The model under review builds one solid part; all positions refer to its coordinate system, in mm. A direction names the side the tool comes from. Give positions to 0.01 mm unless a question says otherwise; leave off trailing zeros. Order: outer loops, then holes, each group sorted by start corner. A loop starts at its lowest first (then second) coordinate and runs counter-clockwise, first axis right, second up. Notation, with made-up numbers: (54.5, 1.25) - (110.5, 1.25) arc R21 cw to (110.5, 20.25) - close; hole circle Ø6 at (39, 53.25). An arc over 180 degrees is marked (long way). Put each result on its own line as item: value.
```python
from build123d import *

# Parameters (mm, degrees)
F1_DEPTH = 6
F0_R     = 1.5
F2_W     = 12.7708302005
F2_H     = 12
F3_DEPTH = 3
F4_R     = 3
F6_DEPTH = 4
F7_D     = 3.3


with BuildPart() as f1:
    # F0 (on Top) → F1 (new body)
    with BuildSketch(Plane.XY):
        with BuildLine():
            ThreePointArc((2.7708302005, -1.15), (-3, 0), (2.7708302005, 1.15))
            Line((2.7708302005, 1.15), (6.7708302005, 1.15))
            Line((6.7708302005, 1.15), (6.7708302005, 6))
            Line((6.7708302005, 6), (-6, 6))
            Line((-6, 6), (-6, 0))
            Line((-6, 0), (-6, -6))
            Line((-6, -6), (6.7708302005, -6))
            Line((6.7708302005, -6), (6.7708302005, -1.15))
            Line((6.7708302005, -1.15), (2.7708302005, -1.15))
        make_face()
    extrude(amount=F1_DEPTH)



with BuildPart() as f1b:
    # F0 (on Top) → F1, piece 2 (new body)
    with BuildSketch(Plane.XY):
        Circle(F0_R)
    extrude(amount=F1_DEPTH)


with BuildPart() as f1_1:
    add(f1.part)

    add(f1b.part)  # F3 merges F1b
    # F2 (on face) → F3 (join)
    with BuildSketch(Plane(origin=(0, 0, 0), x_dir=(1, 0, 0), z_dir=(0, 0, -1))):
        with Locations((0.3854151002, 0)):
            Rectangle(F2_W, F2_H)
    extrude(amount=F3_DEPTH)

    # F4
    f4_edges = [f1_1.edges().sort_by_distance(p)[0] for p in [
        (2.77083, -1.15, 3),
        (2.77083, 1.15, 3),
    ]]
    fillet(f4_edges, radius=F4_R)

    # F5 (on face) → F6 (join)
    with BuildSketch(Plane(origin=(-6, 0, 0), x_dir=(0, -1, 0), z_dir=(-1, 0, 0))):
        with BuildLine():
            Line((-6, -3), (-6, 6))
            Line((-6, 6), (-10, 6))
            ThreePointArc((-10, 6), (-13.1819805153, 4.6819805153), (-14.5, 1.5))
            ThreePointArc((-14.5, 1.5), (-13.1819805153, -1.6819805153), (-10, -3))
            Line((-10, -3), (-6, -3))
        make_face()
        with BuildLine():
            Line((10, 6), (6, 6))
            Line((6, 6), (6, -3))
            Line((6, -3), (10, -3))
            ThreePointArc((10, -3), (13.1819805153, -1.6819805153), (14.5, 1.5))
            ThreePointArc((14.5, 1.5), (13.1819805153, 4.6819805153), (10, 6))
        make_face()
    extrude(amount=-F6_DEPTH)

    # F7 (through all)
    with Locations(Plane(origin=(-6, 0, 0), x_dir=(0, -1, 0), z_dir=(-1, 0, 0))):
        with Locations((-10, 1.5), (10, 1.5)):
            Hole(F7_D / 2)


solid = f1_1.part
```
(1) Take a section at D-D, the plane x = 0. Write out the cut boundary in (y, z).
The answers:
outline: (-6, -3) - (6, -3) - (6, 6) - (3, 6) - (3, 0) - (1.5, 0) - (1.5, 6) - (-1.5, 6) - (-1.5, 0) - (-3, 0) - (-3, 6) - (-6, 6) - close
(2) Take a section at C-C, the plane x = -4. Write out the cut boundary in (y, z).
The answers:
outline: (-10, -3) - (10, -3) arc R4.5 ccw to (10, 6) - (-10, 6) arc R4.5 ccw to start; hole circle Ø3.3 at (-10, 1.5); hole circle Ø3.3 at (10, 1.5)
(3) For faces 1 (the flat face through (6, 1.15, 3)), 2 (the flat face through (-2, -8, 2)), 3 (the flat face through (-2, 8, 3)), list the 3-axis set-ups (+Z, -Z, +X, -X, +Y, -Y) from which the entire face can be reached by the end or side of a thin tool; tool diameter is ignored.
The answers:
face 1: +Z, +X
face 2: +Z, -Z, +X, -Y
face 3: +Z, -Z, +X, +Y
(4) Take a section at B-B, the plane y = -10.75. Write out the cut boundary in (x, z).
The answers:
outline: (-6, -2.94) - (-2, -2.94) - (-2, 0.03) - (-6, 0.03) - close; (-6, 2.97) - (-2, 2.97) - (-2, 5.94) - (-6, 5.94) - close
(5) Take a section at A-A, the plane z = 5.25. Write out the cut boundary in (x, y) (3 decimals).
The answers:
outline: (-6, -12.487) - (-2, -12.487) - (-2, -6) - (6.771, -6) - (6.771, -1.15) - (4.333, -1.15) arc R3 ccw to (2.167, -2.075) arc R3 cw (long way) to (2.167, 2.075) arc R3 ccw to (4.333, 1.15) - (6.771, 1.15) - (6.771, 6) - (-2, 6) - (-2, 12.487) - (-6, 12.487) - close; circle Ø3 at (0, 0)
(6) The part is to be moulded in two halves that separate along X. For faces 4 (the flat face through (6, -1.15, 3)), 5 (the flat face through (2, 0, 0)), 6 (the flat face through (6.771, 1.4, 1.6)), say which applies: pulls with the +X half, pulls with the -X half, needs draft (parallel to the pull), parting line crosses it, or undercut.
The answers:
face 4: needs draft
face 5: undercut
face 6: pulls with the +X half
(7) Wall thickness on L1, parallel to Y at x = 0, z = 3.7; L2, parallel to Z at x = -3.95, y = -10; L3, parallel to Y at x = 0.5, z = 3.25: over which ranges is each line inside the solid? List them lowest first.
The answers:
L1: -6 to -3, -1.5 to 1.5, 3 to 6
L2: -3 to -0.15, 3.15 to 6
L3: -6 to -2.96, -1.41 to 1.41, 2.96 to 6
(8) Clearance check with flat-ended pins moving along their axes: pin 1 Ø2.5 at (x, z) = (4, 3.5) entering from -Y; pin 2 Ø0.7 at (x, z) = (6, 3) entering from +Y; pin 3 Ø4 at (x, z) = (-3.5, -1) entering from +Y; pin 4 Ø4.5 at (y, z) = (10, 1.5) entering from -X. State where each tip first meets the part, or that it passes through.
The answers:
pin 1: y = -6
pin 2: y = 6
pin 3: y = 14.47
pin 4: x = -6
